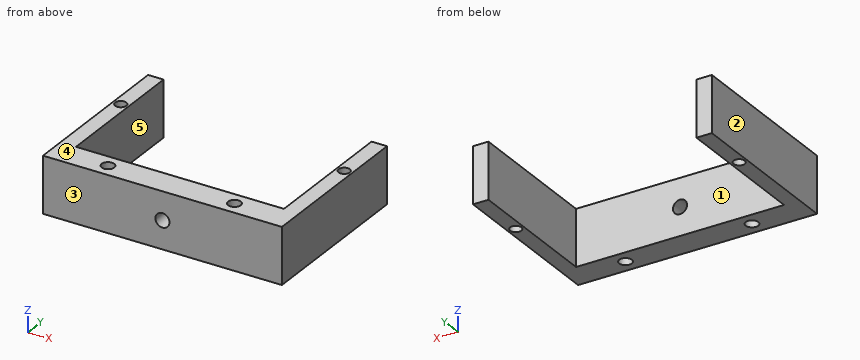
from build123d import *

# Parameters (mm, degrees)
BOSS_EXTRUDE1_DEPTH = 20
SKETCH2_R           = 2.25
CUT_EXTRUDE1_DEPTH  = 20
CUT_EXTRUDE2_REACH  = 22
SKETCH3_R           = 2
CUT_EXTRUDE3_REACH  = 12
SKETCH4_R           = 2.5


with BuildPart() as part:
    # Sketch1 → Boss-Extrude1 (new body)
    with BuildSketch(Plane.XY):
        Polygon((-58.140719223, -46.171804232), (26.859280777, -46.171804232), (26.859280777, 13.828195768), (21.359280777, 13.828195768), (21.359280777, -36.171804232), (-52.640719223, -36.171804232), (-52.640719223, 13.828195768), (-58.140719223, 13.828195768), align=None)
    extrude(amount=BOSS_EXTRUDE1_DEPTH)

    # Sketch2 → Cut-Extrude1 (cut)
    with BuildSketch(Plane(origin=(0, 0, 0), x_dir=(-1, 0, 0), z_dir=(0, 0, -1))):
        with Locations((-6.859280777, -41.171804232)):
            Circle(SKETCH2_R)
        with Locations((38.140719223, -41.171804232)):
            Circle(SKETCH2_R)
    extrude(amount=-CUT_EXTRUDE1_DEPTH, mode=Mode.SUBTRACT)

    # Sketch3 → Cut-Extrude2 (cut, up to next)
    with BuildSketch(Plane.XY.offset(20), mode=Mode.PRIVATE) as cut_extrude2_sk1:
        with Locations((-55.390719223, -6.171804232)):
            Circle(SKETCH3_R)
    cut_extrude2_tool1 = extrude(cut_extrude2_sk1.sketch, amount=-CUT_EXTRUDE2_REACH, mode=Mode.PRIVATE) & part.part
    add(cut_extrude2_tool1.solids().sort_by_distance((-55.390719, -6.171804, 20))[0], mode=Mode.SUBTRACT)
    # Sketch3 → Cut-Extrude2 (cut, up to next)
    with BuildSketch(Plane.XY.offset(20), mode=Mode.PRIVATE) as cut_extrude2_sk2:
        with Locations((24.109280777, -6.171804232)):
            Circle(SKETCH3_R)
    cut_extrude2_tool2 = extrude(cut_extrude2_sk2.sketch, amount=-CUT_EXTRUDE2_REACH, mode=Mode.PRIVATE) & part.part
    add(cut_extrude2_tool2.solids().sort_by_distance((24.109281, -6.171804, 20))[0], mode=Mode.SUBTRACT)

    # Sketch4 → Cut-Extrude3 (cut, up to next)
    with BuildSketch(Plane(origin=(0, -36.171804232, 0), x_dir=(1, 0, 0), z_dir=(0, 1, 0)), mode=Mode.PRIVATE) as cut_extrude3_sk1:
        with Locations((-15.640719223, -10)):
            Circle(SKETCH4_R)
    cut_extrude3_tool1 = extrude(cut_extrude3_sk1.sketch, amount=-CUT_EXTRUDE3_REACH, mode=Mode.PRIVATE) & part.part
    add(cut_extrude3_tool1.solids().sort_by_distance((-15.640719, -36.171804, 10))[0], mode=Mode.SUBTRACT)


solid = part.part
Input: part model. Units: mm. Frame: model coordinates. Face numbers are marked on the shaded views. A direction names the side the tool comes from. Coordinates: 2 decimals unless noted, no trailing zeros. Order: outer loops, then holes, each group sorted by start corner. A loop starts at its lowest first (then second) coordinate and runs counter-clockwise, first axis right, second up. Notation, with made-up numbers: M 13.5,62.25 L 39.5,62.25 A20 cw 39.5,74.25 Z; hole C 78.5,-17 d1. An arc over 180 degrees is marked long. Answer as CSV lines item,"result".
1. Section B-B (y = -26.5). Return the cut outline in (x, z).
Reported:
outline,"M -58.14,0 L -52.64,0 L -52.64,20 L -58.14,20 Z; M 21.36,0 L 26.86,0 L 26.86,20 L 21.36,20 Z"
2. Pull-direction query (X, two-part tool) for the marked faces 1, 2 and 3; classes: released by +X, released by -X, zero draft, split by the parting line, or undercut.
Reported:
face 1,"undercut"
face 2,"released by -X"
face 3,"zero draft"
3. Access query for the marked faces 4 and 5. Directions: +Z, -Z, +X, -X, +Y, -Y. A direction counts if a zero-diameter tool reaches every point of the face in a straight line with its end or side. Return the directions, or none.
Reported:
face 4,"+Z, +X, -X, +Y, -Y"
face 5,"+Z, -Z, +Y"
4. First-contact query: P1, Ø6, axis at x = -18.5, z = 13.5, coming from the +Y side. Flat tip, straight axial feed; report the tip coordinate or a pass-through.
Reported:
P1,"y = -36.17"
5. Material intervals for line 1 (X direction, y = -6, z = 14); line 2 (X direction, y = 11, z = 15.25); line 3 (Y direction, x = -38, z = 10), sorted ascending. Write a range as from..to.
Reported:
line 1,"-58.14..-57.38, -53.4..-52.64, 21.36..22.12, 26.1..26.86"
line 2,"-58.14..-52.64, 21.36..26.86"
line 3,"-46.17..-43.42, -38.93..-36.17"
6. Section D-D (z = 11.5). Return the cut outline in (x, y), then the cut area to 3 significant figures.
Reported:
outline,"M -58.14,-46.17 L -17.64,-46.17 L -17.64,-36.17 L -52.64,-36.17 L -52.64,13.83 L -58.14,13.83 Z; M -13.64,-46.17 L 26.86,-46.17 L 26.86,13.83 L 21.36,13.83 L 21.36,-36.17 L -13.64,-36.17 Z; hole C -55.39,-6.17 d4; hole C -38.14,-41.17 d4.5; hole C 6.86,-41.17 d4.5; hole C 24.11,-6.17 d4"
area,"1,300 mm2"
7. Section A-A (y = -40). Return the cut outline in (x, z).
Reported:
outline,"M -58.14,0 L -40.06,0 L -40.06,20 L -58.14,20 Z; M -36.22,0 L 4.94,0 L 4.94,20 L -36.22,20 Z; M 8.78,0 L 26.86,0 L 26.86,20 L 8.78,20 Z; hole C -15.64,10 d5"
8. Section C-C (x = -37.5). Return the cut outline in (y, z), then the cut area to 3 significant figures.
Reported:
outline,"M -46.17,0 L -43.33,0 L -43.33,20 L -46.17,20 Z; M -39.01,0 L -36.17,0 L -36.17,20 L -39.01,20 Z"
area,"114 mm2"
